```python
from build123d import *
from build123d.topology import SkipClean

# Parameters (mm, degrees)
SKETCH_1_R          = 1.5
EXTRUDE_1_DEPTH     = 17.705
SKETCH_2_R          = 2.5
EXTRUDE_2_DEPTH     = 10
FILLET_1_R          = 1
CUT_EXTRUDE_1_DEPTH = 10
EXTRUDE_START       = 17.795
SKETCH_6_R          = 1.5
EXTRUDE_3_DEPTH     = 17.795
SKETCH_7_R          = 1
EXTRUDE_4_DEPTH     = 2.5


with BuildPart() as part:
    # 草图1 → 凸台-拉伸1 (new body)
    with BuildSketch(Plane.XY):
        Circle(SKETCH_1_R)
    extrude(amount=EXTRUDE_1_DEPTH)

    # 草图2 → 凸台-拉伸2 (add)
    with BuildSketch(Plane.XY.offset(17.705)):
        Circle(SKETCH_2_R)
    extrude(amount=EXTRUDE_2_DEPTH)

    # 圆角1
    fillet_1_edges = [part.edges().sort_by_distance(p)[0] for p in [
        (-1.5, 0, 17.705),
    ]]
    fillet(fillet_1_edges, radius=FILLET_1_R - 0.0001)  # a hair under: the kernel refuses the full size

    # 草图3 → 旋转1 (revolve)
    with SkipClean():  # the faces are left unmerged after this step: merging them gives an invalid solid
        with BuildSketch(Plane(origin=(0, 0, 0), x_dir=(0, 0, -1), z_dir=(1, 0, 0))):
            with BuildLine():
                ThreePointArc((-30.205, 0), (-27.705, -2.5), (-25.205, 0))
                Line((-25.205, 0), (-27.705, 0))
                Line((-27.705, 0), (-30.205, 0))
            make_face()
            with BuildLine():
                Line((-27.705, 0), (-25.205, 0))
                ThreePointArc((-25.205, 0), (-27.705, 2.5), (-30.205, 0))
                Line((-30.205, 0), (-27.705, 0))
            make_face()
        revolve(axis=Axis((0, 0, 0), (0, 0, 1)))
    add(part.part.scale(1), mode=Mode.REPLACE)  # the faces are merged on a copy

    # 草图4 → 切除-拉伸1 (cut)
    with BuildSketch(Plane.XY.offset(30.205)):
        Polygon((-2.5, -1), (0, -1), (2.5, -1), (2.5, -3), (-2.5, -3), align=None)
    extrude(amount=-CUT_EXTRUDE_1_DEPTH, mode=Mode.SUBTRACT)

    # 草图5 → 切除-旋转11 (revolve, cut)
    with BuildSketch(Plane(origin=(0, 0, 0), x_dir=(0, 0, -1), z_dir=(1, 0, 0))):
        with BuildLine():
            Line((-26.25, 0), (-29.16, 0))
            ThreePointArc((-29.16, 0), (-27.705, -1.455), (-26.25, 0))
        make_face()
    revolve(axis=Axis((0, 0, 0), (0, 0, 1)), mode=Mode.SUBTRACT)

    # 草图6 → 凸台-拉伸3 (add)
    with SkipClean():  # the faces are left unmerged after this step: merging them gives an invalid solid
        with BuildSketch(Plane(origin=(0, 0, 0), x_dir=(-1, 0, 0), z_dir=(0, 0, -1)).offset(EXTRUDE_START)):
            Circle(SKETCH_6_R)
        extrude(amount=-EXTRUDE_3_DEPTH)

    # 草图7 → 凸台-拉伸4 (add, symmetric)
    with BuildSketch(Plane(origin=(0, 0, 0), x_dir=(0, 0, -1), z_dir=(1, 0, 0))):
        with BuildLine():
            Line((17.795, -2), (27.795, -2))
            ThreePointArc((27.795, -2), (29.795, 0), (27.795, 2))
            Line((27.795, 2), (17.795, 2))
            Line((17.795, 2), (17.795, -2))
        make_face()
        with Locations((27.795, 0)):
            Circle(SKETCH_7_R, mode=Mode.SUBTRACT)
    extrude(amount=EXTRUDE_4_DEPTH, both=True)


solid = part.part
```
Geometry check sheet. Reference: the model listing, model coordinates, mm. A direction names the side the tool comes from. Coordinates: 2 decimals unless noted, no trailing zeros. Order: outer loops, then holes, each group sorted by start corner. A loop starts at its lowest first (then second) coordinate and runs counter-clockwise, first axis right, second up. Notation, with made-up numbers: (61.25, 76) - (77.25, 76) arc R18 ccw to (77.25, 93) - close; hole circle Ø11 at (68, 53). An arc over 180 degrees is marked (long way). Answer in a Markdown table with one row per item. Add a question column.
1. Section check C-C (z = 15). Enter the section's corners in (x, y), plus the area to 3 significant figures.
2. Draft check along Z on faces 4 (the face through (2.5, 0, -24)), 5 (the face through (0, -2, 20.205)), 6 (the face through (-0.04, 0.3, -28.75)), 7 (the face through (0.035, -0.044, -29.795)). Enter one of: +Z half, -Z half, draft (parallel to the pull), parting line (faces both ways), or undercut.
3. Gauge pin test, flat ends, axial feed: pin 1 Ø1.5 at (x, z) = (-1.5, -14.5) entering from -Y; pin 2 Ø1 at (x, y) = (-1.5, 1.5) entering from -Z; pin 3 Ø2.5 at (x, z) = (0, 23.5) entering from -Y. Record the tip position at first contact, or that the pin passes through.
4. Access from +Z, -Z, +X, -X, +Y, -Y to the whole of each face (thin tool, end or side, straight path). Record for faces 1 (the face through (2, 0, -17.795)), 2 (the face through (0, -1, 25)), 3 (the face through (0, 2, -23)).
5. Section check D-D (z = 22.5). Enter the section's corners in (x, y), plus the area to 3 significant figures.
6. Section check A-A (y = 0). Give the number of separate pieces and of enclosed holes in the cut face, plus the area to 3 significant figures.
7. Material ranges on L1, parallel to Z at x = 0.4, y = 0.35; L2, parallel to Z at x = 1.9, y = -0.4 (3 decimals); L3, parallel to Y at x = -2, z = -22, recorded low to high. Write a range as [from, to].
Data:
| question | item | result |
|---|---|---|
| 1 | outline | circle Ø3 at (0, 0) |
| 1 | area | 7.07 mm² |
| 2 | face 4 | draft |
| 2 | face 5 | +Z half |
| 2 | face 6 | undercut |
| 2 | face 7 | -Z half |
| 3 | pin 1 | stops at y = -1.3 |
| 3 | pin 2 | stops at z = -29.53 |
| 3 | pin 3 | stops at y = -1 |
| 4 | face 1 | none |
| 4 | face 2 | +Z, +X, -X, -Y |
| 4 | face 3 | -Z, +X, -X, +Y |
| 5 | outline | (-2.29, -1) - (2.29, -1) arc R2.5 ccw (long way) to start |
| 5 | area | 14.7 mm² |
| 6 | separate pieces | 2 |
| 6 | enclosed holes | 1 |
| 6 | area | 210 mm² |
| 7 | L1 | z = [-29.76, -28.73], [-26.86, 26.35], [29.06, 30.15] |
| 7 | L2 | z = [-29.755, -28.712], [-26.878, -17.795], [17.535, 29.28] |
| 7 | L3 | y = [-2, 2] |
